Work out the finished part from the listing and answer in its coordinate system (mm). A direction names the side the tool comes from. Round coordinates to 2 decimals unless told otherwise and drop trailing zeros. Answer in a Markdown table with one row per item.
Autodesk Inventor part; units mm, degrees
ref_plane "YZ Plane" through (0, 0, 0) normal (1, 0, 0) x (0, 1, 0)
ref_plane "XZ Plane" through (0, 0, 0) normal (0, 1, 0) x (-1, 0, 0)
ref_plane "XY Plane" through (0, 0, 0) normal (0, 0, 1) x (1, 0, 0)
sketch "Sketch5" plane through (0, 0, 0) normal (0, 1, 0) x (-1, 0, 0)
  circle A0 centre (0, 0) radius 9.975
  dimension "d20" = 19.95
extrude "Extrusion4" add sketch "Sketch5" against normal blind 2.5
sketch "Sketch6" plane through (0, -2.5, 0) normal (0, -1, 0) x (1, 0, 0)
  circle A0 centre (0, 0) radius 4.5
  dimension "d23" = 9
extrude "Extrusion5" add sketch "Sketch6" along normal blind 2
sketch "Sketch7" plane through (0, -4.5, 0) normal (0, -1, 0) x (1, 0, 0)
  circle A0 centre (0, 0) radius 2.925
  dimension "d26" = 5.85
extrude "Extrusion6" cut sketch "Sketch7" against normal blind 3.6
sketch "Sketch8" plane through (0, 0, 0) normal (0, 1, 0) x (1, 0, 0)
  circle A0 centre (0, 0) radius 1.75
  dimension "d29" = 3.5
extrude "Extrusion7" cut sketch "Sketch8" against normal through all
sketch "Sketch9" plane through (0, 0, 0) normal (0, 1, 0) x (1, 0, 0)
  circle A0 centre (0, 0) radius 7
  point P0 (-7, 0)
  point P1 (7, 0)
  point P2 (0, 7)
  point P3 (0, -7)
  dimension "d32" = 14
hole "Hole2" at (-7, 0, 0) at (7, 0, 0) at (0, 0, -7) at (0, 0, 7) direction (0, -1, 0) diameter 1.567 end through all
chamfer "Chamfer2" distance 0.1 angle 45 3 edges at (9.975, 0, 0) (9.975, -2.5, 0) (-4.5, -4.5, 0)
properties part number "Top Horn" material "Aluminum 6061"
1) Each of these flat-tipped pins is pushed along its axis until it touches: pin 1 (1.3 mm diameter, centred on x = 0, z = 7, fed in from +Y); pin 2 (1 mm diameter, centred on y = -4, z = 0.5, fed in from +X); pin 3 (1 mm diameter, centred on x = -2, y = -2, fed in from +Z); pin 4 (1.8 mm diameter, centred on x = 0, z = -7, fed in from -Y). Where does it stop, or does it pass through?
Filled in:
| item | result |
|---|---|
| pin 1 | passes through |
| pin 2 | stops at x = 4.5 |
| pin 3 | stops at z = 9.86 |
| pin 4 | stops at y = -2.5 |
2) Find the intervals of material crossed by probe 1 along Z at (x, y) = (0, -1.75) (1 decimal); probe 2 along Y at (x, z) = (3, -6); probe 3 along Z at (x, y) = (1.75, -1.6), in increasing order. Write a range as from..to.
Filled in:
| item | result |
|---|---|
| probe 1 | z = -10..-7.8, -6.2..-2.9, 2.9..6.2, 7.8..10 |
| probe 2 | y = -2.5..0 |
| probe 3 | z = -9.82..-2.34, 2.34..9.82 |
3) Which of the six approach directions +Z, -Z, +X, -X, +Y, -Y give full straight-line access (tool end or side, diameter ignored) to faces 1 (the face through (2, -0.9, 0)), 2 (the face through (0.3, -1.268, 7.724))?
Filled in:
| item | result |
|---|---|
| face 1 | -Y |
| face 2 | +Y, -Y |
4) Find section A-A, the plane z = 0. Give the number of separate pieces and of enclosed holes in the cut face, then the cut area to 3 significant figures.
Filled in:
| item | result |
|---|---|
| separate pieces | 4 |
| enclosed holes | 0 |
| area | 35.8 mm^2 |
5) The mould has two halves that part along X. Classify faces 3 (the face through (-9.514, -1.234, 2.996)), 4 (the face through (-0.634, -2.725, -2.855)), 5 (the face through (-4.3, -2.5, -2.1)): released by +X, released by -X, zero draft, split by the parting line, or undercut.
Filled in:
| item | result |
|---|---|
| face 3 | split by the parting line |
| face 4 | undercut |
| face 5 | zero draft |
